Geometry check sheet. Reference: the model listing, model coordinates, mm. Face numbers are marked on the shaded views. Give positions to 0.01 mm unless a question says otherwise; leave off trailing zeros. Loops run counter-clockwise (first coordinate to the right, second up) from the corner with the lowest first, then second, coordinate; pieces in that order, holes last. Notation, with made-up numbers: (-21.75, 50) -> (7.25, 50) arc R25 ccw to (7.25, 72) -> close; hole circle Ø4 at (62, 57.5). An arc over 180 degrees is marked (long way). Answer as a JSON object with one key per item and string values.
Autodesk Inventor part; units mm, degrees
ref_plane "YZ Plane" through (0, 0, 0) normal (1, 0, 0) x (0, 1, 0)
ref_plane "XZ Plane" through (0, 0, 0) normal (0, 1, 0) x (-1, 0, 0)
ref_plane "XY Plane" through (0, 0, 0) normal (0, 0, 1) x (1, 0, 0)
sketch "Sketch1" plane through (0, 0, 0) normal (0, 1, 0) x (-1, 0, 0)
  line L0 (0, 0) -> (40, 0)
  line L1 (40, 0) -> (40, -40)
  line L2 (40, -40) -> (0, -40)
  line L3 (0, -40) -> (0, 0)
  dimension "d0" = 40
  dimension "d1" = 40
extrude "Extrusion1" add sketch "Sketch1" along normal blind 5
sketch "Sketch2" plane through (0, 5, 0) normal (0, 1, 0) x (1, 0, 0)
  line L0 (-40, 0) -> (0, 0)
  line L1 (0, 0) -> (0, 40)
  line L2 (0, 40) -> (-40, 40)
  line L3 (-40, 40) -> (-40, 0)
  point P0 (-4, 4)
  point P1 (-4, 36)
  point P2 (-36, 36)
  point P3 (-36, 4)
  dimension "d4" = 4
  dimension "d6" = 4
  dimension "d7" = 4
  dimension "d8" = 4
  dimension "d9" = 4
  dimension "d10" = 4
  dimension "d11" = 4
  dimension "d12" = 4
hole "Hole1" at (-4, 5, -4) at (-4, 5, -36) at (-36, 5, -36) at (-36, 5, -4) direction (0, -1, 0) diameter 4.3 end through all countersink diameter 6 countersink angle 90
sketch "Sketch3" plane through (0, 5, 0) normal (0, 1, 0) x (1, 0, 0)
  circle A0 centre (-20, 20) radius 17.5
  line L0 (-40, 0) -> (0, 0)
  line L1 (-40, 40) -> (-40, 0)
  dimension "d21" = 20
  dimension "d22" = 20
  dimension "d23" = 35
extrude "Extrusion2" cut sketch "Sketch3" against normal blind 0.1
properties part number "Filter"
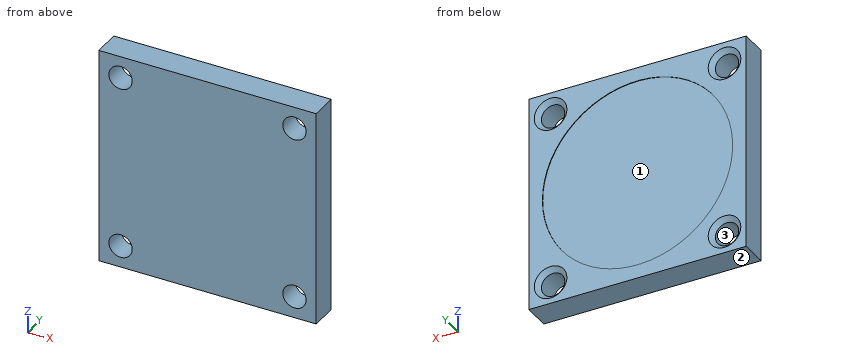
1) Section check A-A on x = -20. Record the cut outline in (y, z), plus the area to 4 significant figures.
Geometry check:
{"outline": "(0, -40) -> (5, -40) -> (5, -37.5) -> (4.9, -37.5) -> (4.9, -2.5) -> (5, -2.5) -> (5, 0) -> (0, 0) -> close", "area": "196.5 mm2"}
2) Material ranges on line 1 along X through (y, z) = (2.15, -36); line 2 along X through (y, z) = (4.95, -20), recorded low to high. Write a range as from..to.
Geometry check:
{"line 1": "x = -40..-38.15, -33.85..-6.15, -1.85..0", "line 2": "x = -40..-37.5, -2.5..0"}
3) Depth check by flat-ended pin: P1, Ø1.5, axis at x = -24, z = -13.5, coming from the +Y side; P2, Ø3.5, axis at x = -36, z = -4, coming from the -Y side; P3, Ø5, axis at x = -4, z = -4, coming from the +Y side. Enter the tip coordinate at first touch or a pass-through.
Geometry check:
{"P1": "stops at y = 4.9", "P2": "passes through", "P3": "stops at y = 4.5"}
4) Section check C-C on z = -4. Record the cut outline in (x, y), plus the area to 3 significant figures.
Geometry check:
{"outline": "(-40, 0) -> (-38.15, 0) -> (-38.15, 4.15) -> (-39, 5) -> (-40, 5) -> close; (-33.85, 0) -> (-6.15, 0) -> (-6.15, 4.15) -> (-7, 5) -> (-12.91, 5) -> (-12.91, 4.9) -> (-27.09, 4.9) -> (-27.09, 5) -> (-33, 5) -> (-33.85, 4.15) -> close; (-1.85, 0) -> (0, 0) -> (0, 5) -> (-1, 5) -> (-1.85, 4.15) -> close", "area": "154 mm2"}
5) Section check D-D on x = -36. Record the cut outline in (y, z).
Geometry check:
{"outline": "(0, -40) -> (5, -40) -> (5, -39) -> (4.15, -38.15) -> (0, -38.15) -> close; (0, -33.85) -> (4.15, -33.85) -> (5, -33) -> (5, -27.09) -> (4.9, -27.09) -> (4.9, -12.91) -> (5, -12.91) -> (5, -7) -> (4.15, -6.15) -> (0, -6.15) -> close; (0, -1.85) -> (4.15, -1.85) -> (5, -1) -> (5, 0) -> (0, 0) -> close"}
6) Draft check along X on the marked faces 1, 2 and 3. Enter one of: pulls with the +X half, pulls with the -X half, needs draft (parallel to the pull), parting line crosses it, or undercut.
Geometry check:
{"face 1": "undercut", "face 2": "needs draft", "face 3": "undercut"}
7) Section check B-B on y = 2.1. Record the cut outline in (x, z), plus the area to 3 significant figures.
Geometry check:
{"outline": "(-40, -40) -> (0, -40) -> (0, 0) -> (-40, 0) -> close; hole circle Ø4.3 at (-36, -36); hole circle Ø4.3 at (-36, -4); hole circle Ø4.3 at (-4, -36); hole circle Ø4.3 at (-4, -4)", "area": "1,540 mm2"}
